Verification items for this drawing (mm, ordinates from the low corner). A direction names the side the tool comes from. Coordinates: 2 decimals unless noted, no trailing zeros. Loops run counter-clockwise (first coordinate to the right, second up) from the corner with the lowest first, then second, coordinate; pieces in that order, holes last. Notation, with made-up numbers: M -39.5,31 L 13.5,31 A24 ccw 13.5,68 Z; hole C 85.5,-2.5 d1. An arc over 180 degrees is marked long. Return JSON: item names as keys, results as strings.
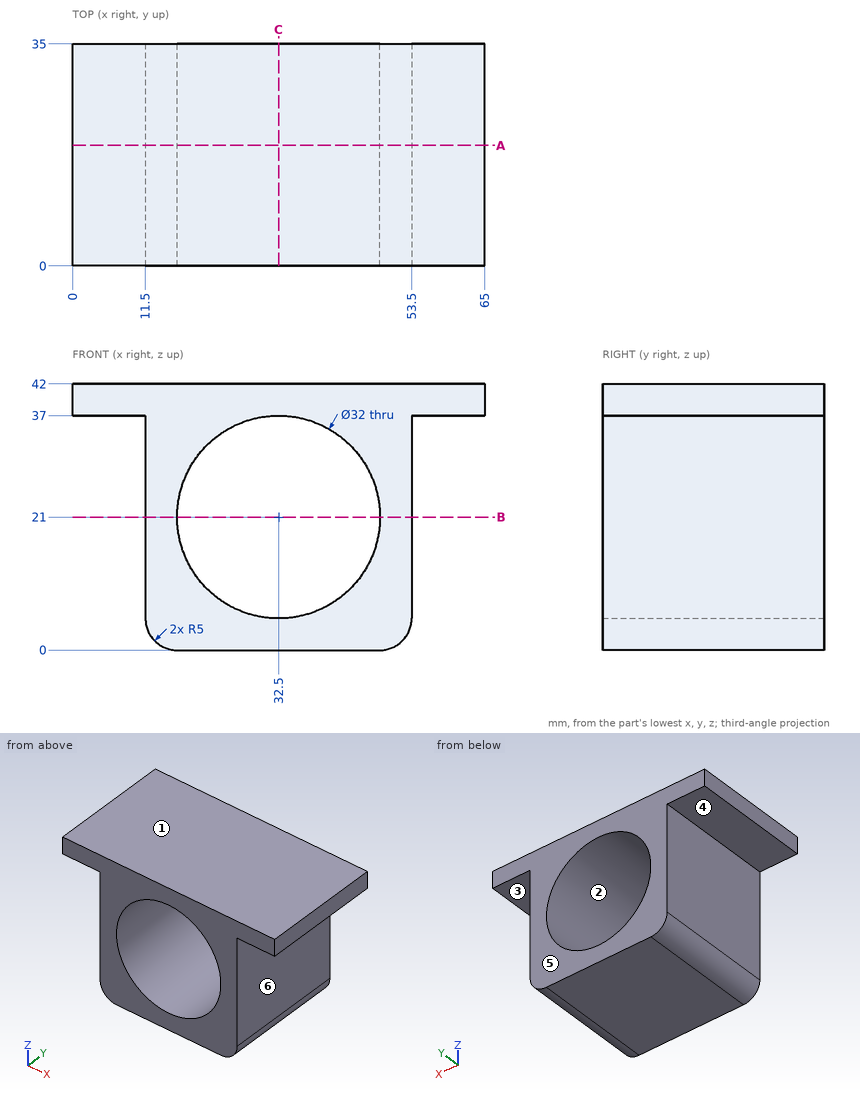
1) Section check C-C on x = 32.5. Record the cut outline in (y, z).
Answers:
{"outline": "M 0,0 L 35,0 L 35,5 L 0,5 Z; M 0,37 L 35,37 L 35,42 L 0,42 Z"}
2) Go/stop test with flat-tipped pins: pin 1 Ø10 at (x, z) = (30, 32) entering from -Y; pin 2 Ø1.5 at (y, z) = (28.5, 19.5) entering from -X; pin 3 Ø2 at (y, z) = (11.5, 11.5) entering from +X; pin 4 Ø6 at (x, y) = (59.5, 15) entering from -Z. Record where each tip stops, or that it passes through.
Answers:
{"pin 1": "y = 0", "pin 2": "x = 11.5", "pin 3": "x = 53.5", "pin 4": "z = 37"}
3) Scan lines: line 1 along X through (y, z) = (17, 21); line 2 along Z through (x, y) = (57.5, 33.5); line 3 along Z through (x, y) = (32, 16). Record each from-to range of solid material in increasing order. Write a range as [from, to].
Answers:
{"line 1": "[11.5, 16.5], [48.5, 53.5]", "line 2": "[37, 42]", "line 3": "[0, 5.01], [36.99, 42]"}
4) Draft check along Z on the marked faces 1, 2 and 3. Enter one of: +Z half, -Z half, draft (parallel to the pull), parting line (faces both ways), or undercut.
Answers:
{"face 1": "+Z half", "face 2": "undercut", "face 3": "-Z half"}
5) Set-up check for the marked faces 4, 5 and 6: record each of +Z, -Z, +X, -X, +Y, -Y from which the full face is reachable in a straight line by a thin tool's end or side.
Answers:
{"face 4": "-Z, -X, +Y, -Y", "face 5": "+Z, -Z, +X, -X, +Y", "face 6": "-Z, +X, +Y, -Y"}
6) Section check B-B on z = 21. Record the cut outline in (x, y), then the cut area to 3 significant figures.
Answers:
{"outline": "M 11.5,0 L 16.5,0 L 16.5,35 L 11.5,35 Z; M 48.5,0 L 53.5,0 L 53.5,35 L 48.5,35 Z", "area": "350 mm²"}
7) Section check A-A on y = 19. Record the cut outline in (x, z).
Answers:
{"outline": "M 0,37 L 11.5,37 L 11.5,5 A5 ccw 16.5,0 L 48.5,0 A5 ccw 53.5,5 L 53.5,37 L 65,37 L 65,42 L 0,42 Z; hole C 32.5,21 d32"}
